from build123d import *

# Parameters (mm, degrees)
F0_W     = 0.001
F0_H     = 60
F1_DEPTH = 2


with BuildPart() as f1:
    # F0 (on Top) → F1 (new body)
    with BuildSketch(Plane.XY):
        Polygon((-409.5329046249, 489.3550023332), (-409.5329046249, 703.2591700554), (-439.5329046249, 675.5668623631), (-439.5329046249, 634.7396177178), (-439.5329046249, 219.3550023332), (-439.5329046249, 189.3550023332), (-439.5329046249, -93.071404538), (-409.5329046249, -63.071404538), (-409.5329046249, -20.6449976668), (-409.5329046249, 189.3550023332), (-409.5329046249, 279.3550023332), (-409.5329046249, 399.3550023332), (-409.5329046249, 459.3550023332), align=None)
        Polygon((-187.1064977537, 489.3550023332), (-409.5329046249, 489.3550023332), (-409.5329046249, 459.3550023332), (-199.5329046249, 459.3550023332), (-157.1064977537, 459.3550023332), align=None)
        Polygon((-439.5329046249, 634.7396177178), (-439.5329046249, 675.5668623631), (-499.5329046249, 620.1822469785), (-499.5329046249, 579.3550023332), align=None)
        Polygon((-499.5329046249, 579.3550023332), (-499.5329046249, 620.1822469785), (-529.5329046249, 592.4899392862), (-529.5329046249, 551.6626946409), align=None)
        Polygon((-157.1064977537, 459.3550023332), (-199.5329046249, 459.3550023332), (-139.5329046249, 399.3550023332), (40.4670953751, 219.3550023332), (-44.3857183673, 219.3550023332), (-349.5319046249, 219.3550023332), (-349.5329046249, 219.3550023332), (-349.5329046249, 189.3550023332), (-319.5329046249, 189.3550023332), (112.8935022463, 189.3550023332), align=None)
        Polygon((-439.5329046249, 189.3550023332), (-439.5329046249, 219.3550023332), (-889.5329046249, 219.3550023332), (-922.0329046249, 189.3550023332), align=None)
        Polygon((-499.5329046249, 459.3550023332), (-499.5329046249, 579.3550023332), (-529.5329046249, 551.6626946409), (-529.5329046249, 489.3550023332), (-597.0329046249, 489.3550023332), (-629.5329046249, 459.3550023332), align=None)
        Polygon((-224.3857183673, 399.3550023332), (-349.5329046249, 399.3550023332), (-349.5329046249, 279.3550023332), (-349.5319046249, 279.3550023332), (-104.3857183673, 279.3550023332), align=None)
        Polygon((-922.0329046249, 189.3550023332), (-889.5329046249, 219.3550023332), (-933.7624196573, 219.3550023332), (-966.2624196573, 189.3550023332), align=None)
        Polygon((-933.7624196573, 219.3550023332), (-889.5329046249, 219.3550023332), (-824.5329046249, 279.3550023332), (-868.7624196573, 279.3550023332), align=None)
        Polygon((-597.0329046249, 489.3550023332), (-641.2624196573, 489.3550023332), (-673.7624196573, 459.3550023332), (-629.5329046249, 459.3550023332), align=None)
        with Locations((-349.5324046249, 249.3550023332)):
            Rectangle(F0_W, F0_H)
        Polygon((-319.5329046249, 26.928595462), (-319.5329046249, 189.3550023332), (-349.5329046249, 189.3550023332), (-349.5329046249, 39.3550023332), (-349.5329046249, -3.071404538), align=None)
        Polygon((-694.5329046249, 399.3550023332), (-824.5329046249, 279.3550023332), (-499.5329046249, 279.3550023332), (-499.5329046249, 399.3550023332), align=None)
        Polygon((-868.7624196573, 279.3550023332), (-824.5329046249, 279.3550023332), (-694.5329046249, 399.3550023332), (-738.7624196573, 399.3550023332), align=None)
        Polygon((-694.5329046249, 399.3550023332), (-629.5329046249, 459.3550023332), (-673.7624196573, 459.3550023332), (-738.7624196573, 399.3550023332), align=None)
        Polygon((-349.5329046249, 39.3550023332), (-409.5329046249, -20.6449976668), (-409.5329046249, -63.071404538), (-349.5329046249, -3.071404538), align=None)
    extrude(amount=F1_DEPTH)


solid = f1.part
Check sheet for the modelled part. Datum: model origin and axes. Units: mm. A direction names the side the tool comes from. Round coordinates to 2 decimals unless told otherwise and drop trailing zeros. Order: outer loops, then holes, each group sorted by start corner. A loop starts at its lowest first (then second) coordinate and runs counter-clockwise, first axis right, second up.
(1) Scan lines: probe 1 along Y at (x, z) = (-289, 0.2) (3 decimals); probe 2 along X at (y, z) = (552.5, 1.4); probe 3 along X at (y, z) = (64, 0.9). Record each from-to range of solid material in increasing order.
(2) Draft check along Y on faces 1 (the flat face through (-662.488, 428.935, 0.986)), 2 (the flat face through (-380.37, -33.91, 0.99)), 3 (the flat face through (-801.487, 341.455, 0.986)), 4 (the flat face through (-429, 307, 0)). Enter one of: pulls with the +Y half, pulls with the -Y half, needs draft (parallel to the pull), parting line crosses it, or undercut.
(3) Go/stop test with flat-tipped pins: P1, Ø1, axis at y = 236.5, z = 1, coming from the +X side; P2, Ø1, axis at x = -619.5, z = 0.5, coming from the +Y side (3 decimals); P3, Ø0.6, axis at x = -648, z = 1, coming from the -Y side (3 decimals). Record where each tip stops, or that it passes through.
(4) Cross-section at D-D, the plane x = -367. Enter the section's corners in (y, z) (1 decimal).
(5) Cross-section at A-A, the plane y = 540.5. Enter the section's corners in (x, z).
(6) Cross-section at C-C, the plane z = 1.55. State how many separate pieces and enclosed holes the cut face has, and give its area (3 significant figures).
(7) Cross-section at B-B, the plane x = -583. Enter the section's corners in (y, z) (3 decimals).
(8) Access from +Z, -Z, +X, -X, +Y, -Y to the whole of each face (thin tool, end or side, straight path). Record for faces 5 (the flat face through (-163.55, 338.52, 0.99)), 6 (the flat face through (-468.69, 648.65, 0.99)).
Check sheet entries:
1. probe 1: y = 189.355 to 219.355, 279.355 to 399.355, 459.355 to 489.355
1. probe 2: x = -529.53 to -499.53, -439.53 to -409.53
1. probe 3: x = -439.53 to -409.53, -349.53 to -319.53
2. face 1: undercut
2. face 2: pulls with the -Y half
2. face 3: pulls with the +Y half
2. face 4: needs draft
3. P1: stops at x = 66.25
3. P2: stops at y = 489.355
3. P3: stops at y = 189.355
4. outline: (-20.5, 0) - (21.9, 0) - (21.9, 2) - (-20.5, 2) - close; (459.4, 0) - (489.4, 0) - (489.4, 2) - (459.4, 2) - close
5. outline: (-529.53, 0) - (-499.53, 0) - (-499.53, 2) - (-529.53, 2) - close; (-439.53, 0) - (-409.53, 0) - (-409.53, 2) - (-439.53, 2) - close
6. separate pieces: 1
6. enclosed holes: 2
6. area: 152,000 mm2
7. outline: (189.355, 0) - (219.355, 0) - (219.355, 2) - (189.355, 2) - close; (279.355, 0) - (399.355, 0) - (399.355, 2) - (279.355, 2) - close; (459.355, 0) - (489.355, 0) - (489.355, 2) - (459.355, 2) - close
8. face 5: +Z, -Z
8. face 6: +Z, -Z, -X, +Y
